The listing builds one solid part. Answer for the finished solid, in the listing's coordinates (mm). Face numbers are marked on the shaded views. A direction names the side the tool comes from. Give positions to 0.01 mm unless a question says otherwise; leave off trailing zeros. Write each loop counter-clockwise with the first axis right and the second up, starting at its lowest first coordinate (ties: lowest second). Pieces come first, ordered by that corner, then holes. Notation, with made-up numbers: (31.25, -15) - (73.25, -15) arc R25 ccw to (73.25, 15) - close; hole circle Ø11 at (-15, -27.5). An arc over 180 degrees is marked (long way). Answer in a Markdown table with one row per item. Add a question column.
Autodesk Inventor part; units mm, degrees
ref_plane "YZ Plane" through (0, 0, 0) normal (1, 0, 0) x (0, 1, 0)
ref_plane "XZ Plane" through (0, 0, 0) normal (0, 1, 0) x (-1, 0, 0)
ref_plane "XY Plane" through (0, 0, 0) normal (0, 0, 1) x (1, 0, 0)
sketch "Sketch1" plane through (0, 0, 0) normal (0, 0, 1) x (1, 0, 0)
  line L0 (-33.6112, 18.3384) -> (17.1888, 18.3384)
  line L1 (17.1888, 18.3384) -> (17.1888, -19.7616)
  line L2 (17.1888, -19.7616) -> (-33.6112, -19.7616)
  line L3 (-33.6112, -19.7616) -> (-33.6112, 18.3384)
  point P0 (0, 0)
  dimension "d0" = 50.8
  dimension "d1" = 38.1
extrude "Extrusion1" add sketch "Sketch1" along normal blind 31.75
sketch "Sketch2" plane through (0, 0, 31.75) normal (0, 0, 1) x (1, 0, 0)
  line L0 (17.1888, 18.3384) -> (-33.6112, 18.3384)
  line L1 (17.1888, -19.7616) -> (17.1888, 18.3384)
  line L2 (-33.6112, 18.3384) -> (17.1888, 18.3384)
  line L3 (17.1888, 18.3384) -> (17.1888, -7.0616)
  line L4 (17.1888, -7.0616) -> (-33.6112, -7.0616)
  line L5 (-33.6112, -7.0616) -> (-33.6112, 18.3384)
  line L6 (17.1888, -19.7616) -> (-33.6112, -19.7616)
  point P0 (0, 0)
  dimension "d4" = 12.7
extrude "Extrusion2" cut sketch "Sketch2" against normal blind 12.7
sketch "Sketch3" plane through (0, 0, 19.05) normal (0, 0, 1) x (1, 0, 0)
  line L0 (-33.6112, 18.3384) -> (17.1888, 18.3384)
  line L1 (-20.9112, 18.3384) -> (4.4888, 18.3384)
  line L2 (4.4888, 18.3384) -> (4.4888, -0.7116)
  line L3 (4.4888, -0.7116) -> (-20.9112, -0.7116)
  line L4 (-20.9112, -0.7116) -> (-20.9112, 18.3384)
  line L5 (17.1888, 18.3384) -> (17.1888, -7.0616)
  point P0 (0, 0)
  dimension "d7" = 25.4
  dimension "d8" = 12.7
  dimension "d9" = 19.05
extrude "Extrusion3" cut sketch "Sketch3" against normal blind 12.7
properties part number "Figure 7_27_6"
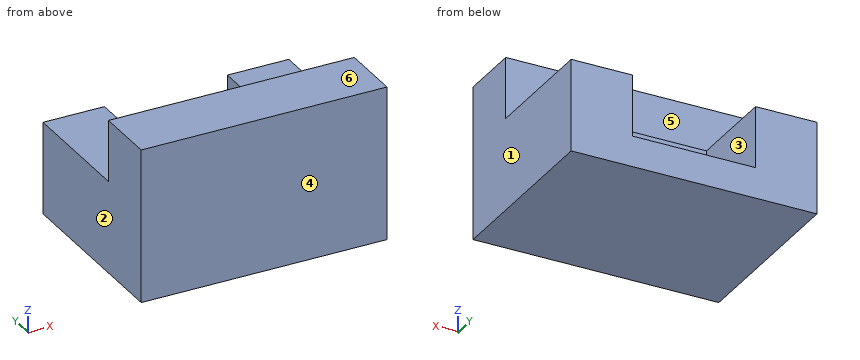
1. The mould has two halves that part along X. Classify the marked faces 1, 2, 3 and 4: +X half, -X half, draft (parallel to the pull), parting line (faces both ways), or undercut.
2. Section C-C (y = -4.5) is taken. Give the vertices of the cut face in (x, z), and give its area (3 significant figures).
3. Straight lines are drawn through the part: L1, parallel to Z at x = 11, y = 7.5; L2, parallel to Y at x = -10.5, z = 16; L3, parallel to Y at x = 15, z = 25. For each, find the intervals that lie inside material, in ascending order. Write a range as [from, to].
4. Section D-D (x = 8) is taken. Give the vertices of the cut face in (y, z), and give its area (3 significant figures).
5. Section B-B (z = 18) is taken. Give the vertices of the cut face in (x, y).
6. A tool of negligible diameter and unlimited length cuts with its end or side. For the marked faces 5 and 6, from which of +Z, -Z, +X, -X, +Y, -Y can it reach the whole face along a straight path? Write none if from no direction.
7. Section A-A (x = -19.5) is taken. Give the vertices of the cut face in (y, z).
8. Given pin 1 Ø12 at (x, y) = (-22, 12) entering from +Z; pin 2 Ø10 at (x, z) = (-9, 24) entering from +Y, each flat-ended and moving along its own axis, determine where each tip first touches the part or whether it passes through.
Geometry check:
| question | item | result |
|---|---|---|
| 1 | face 1 | +X half |
| 1 | face 2 | -X half |
| 1 | face 3 | undercut |
| 1 | face 4 | draft |
| 2 | outline | (-33.61, 0) - (17.19, 0) - (17.19, 19.05) - (-33.61, 19.05) - close |
| 2 | area | 968 mm² |
| 3 | L1 | [0, 19.05] |
| 3 | L2 | [-19.76, -0.71] |
| 3 | L3 | [-19.76, -7.06] |
| 4 | outline | (-19.76, 0) - (18.34, 0) - (18.34, 19.05) - (-7.06, 19.05) - (-7.06, 31.75) - (-19.76, 31.75) - close |
| 4 | area | 887 mm² |
| 5 | outline | (-33.61, -19.76) - (17.19, -19.76) - (17.19, 18.34) - (4.49, 18.34) - (4.49, -0.71) - (-20.91, -0.71) - (-20.91, 18.34) - (-33.61, 18.34) - close |
| 6 | face 5 | +Z, +X, -X, +Y |
| 6 | face 6 | +Z, +X, -X, +Y, -Y |
| 7 | outline | (-19.76, 0) - (18.34, 0) - (18.34, 6.35) - (-0.71, 6.35) - (-0.71, 19.05) - (-7.06, 19.05) - (-7.06, 31.75) - (-19.76, 31.75) - close |
| 8 | pin 1 | z = 19.05 |
| 8 | pin 2 | y = -0.71 |
